Part model, mm, in its own coordinate system. A direction names the side the tool comes from. Round coordinates to 2 decimals unless told otherwise and drop trailing zeros. Loops run counter-clockwise (first coordinate to the right, second up) from the corner with the lowest first, then second, coordinate; pieces in that order, holes last. Notation, with made-up numbers: (-0.5, 14) -> (54.5, 14) arc R29 cw to (54.5, 48) -> close; hole circle Ø2 at (-29, 77.5). An arc over 180 degrees is marked (long way). Use a Markdown table: item, result. Add a question column.
Item 1: Flat gauge pins, fed straight in: pin 1 (2 mm diameter, centred on x = 0.5, z = 32.5, fed in from -Y); pin 2 (3.5 mm diameter, centred on y = -39.23, z = 96.29, fed in from -X); pin 3 (1.5 mm diameter, centred on x = 1.5, y = -72.5, fed in from +Z). Where does each tip first touch, or does it go through?
Item 2: Cut at D-D, the plane y = -136. List the corners of the cut face in (x, z).
Item 3: Cut at A-A, the plane z = 58.5. List the corners of the cut face in (x, y), plus the area to 3 significant figures.
Item 4: Probe line 1 (Y direction, x = 1.55, z = 67.5); line 2 (Z direction, x = 1, y = -125.5); line 3 (Z direction, x = 2.4, y = -58.5). List the from-to ranges inside material, lowest first. Write a range as [from, to].
Item 5: Cut at B-B, the plane y = -99. List the corners of the cut face in (x, z), plus the area to 3 significant figures.
Item 6: Cut at C-C, the plane x = 0.6. State how many separate pieces and enclosed holes the cut face has, plus the area to 3 significant figures.
Item 7: Which spindle directions (+Z, -Z, +X, -X, +Y, -Y) get a long thin tool onto all of the face, cutting with end or side? Do faces 4 (the face through (2, -186.521, 27)), 5 (the face through (2.03, -120.35, 106.77)), 6 (the face through (2, -190.521, 120)), 7 (the face through (2, -133, 10.903)), 8 (the face through (2, -188, 104.903)). Say none if no direction does.
Item 8: Two-plate mould, pull along Z, no slides. Class faces 1 (the face through (2, -186.521, 89)), 2 (the face through (2.03, -91.6, 151.05)), 3 (the face through (2, -186.521, 151)): pulls with the +Z half, pulls with the -Z half, needs draft (parallel to the pull), parting line crosses it, or undercut.
```python
from build123d import *

# Parameters (mm, degrees)
AUFSATZ_LINEAR_AUSTRAGEN1_DEPTH      = 4
SKIZZE1_9_R                          = 10
SCHNITT_LINEAR_AUSTRAGEN1_DEPTH      = 6
F_4_1_4_1_DURCHMESSER_BOHRUNG1_D     = 4.1
F_4_1_4_1_DURCHMESSER_BOHRUNG1_DEPTH = 20
F_4_1_4_1_DURCHMESSER_BOHRUNG1_TIP   = 1.231764269
FASE1_SIZE                           = 1
SCHNITT_LINEAR_AUSTRAGEN2_DEPTH      = 251.325290812
SCHNITT_LINEAR_AUSTRAGEN2_DEPTH_BACK = 10
F_4_8_4_8_DURCHMESSER_BOHRUNG1_D     = 4.8
F_4_8_4_8_DURCHMESSER_BOHRUNG1_DEPTH = 4
F_4_8_4_8_DURCHMESSER_BOHRUNG1_TIP   = 1.442065486
SKIZZE21_R                           = 37.5
SCHNITT_LINEAR_AUSTRAGEN3_DEPTH      = 251.325290812
DURCHGANGSLOCH_F_R_M41_D             = 4.5
KREISMUSTER1_COUNT                   = 6
M3_GEWINDEBOHRUNG1_D                 = 2.5
M3_GEWINDEBOHRUNG1_DEPTH             = 8.5
M3_GEWINDEBOHRUNG1_TIP               = 0.751075774
SCHNITT_LINEAR_AUSTRAGEN4_DEPTH      = 251.325290812
SCHNITT_LINEAR_AUSTRAGEN5_DEPTH      = 251.325290812
VERRUNDUNG1_R                        = 6
SKIZZE31_W                           = 4
SKIZZE31_H                           = 30
AUFSATZ_LINEAR_AUSTRAGEN2_DEPTH      = 4


with BuildPart() as part:
    # Skizze1 → Aufsatz-Linear austragen1 (new body)
    with BuildSketch(Plane(origin=(0, 0, 0), x_dir=(0, 0, -1), z_dir=(1, 0, 0))):
        with BuildLine():
            Line((-120.903454086, -13.395859459), (-120.903454086, -24.075118314))
            ThreePointArc((-120.903454086, -24.075118314), (-140.766673303, -45.238586838), (-150.337818424, -72.639919993))
            Line((-150.337818424, -72.639919993), (-166.903454086, -186.520744783))
            Line((-166.903454086, -186.520744783), (-10.903454086, -186.520744783))
            Line((-10.903454086, -186.520744783), (-1.903454086, -186.520744783))
            Line((-1.903454086, -186.520744783), (-1.903454086, -81.52074478))
            ThreePointArc((-1.903454086, -81.52074478), (-41.654250272, -12.960552248), (-120.903454086, -13.395859459))
        make_face()
    extrude(amount=AUFSATZ_LINEAR_AUSTRAGEN1_DEPTH)

    # Skizze1_9 → Schnitt-Linear austragen1 (cut)
    with BuildSketch(Plane(origin=(0, 0, 0), x_dir=(0, 0, -1), z_dir=(1, 0, 0))):
        with Locations((-80.903454086, -81.52074478)):
            Circle(SKIZZE1_9_R)
    extrude(amount=SCHNITT_LINEAR_AUSTRAGEN1_DEPTH, mode=Mode.SUBTRACT)

    # 4.1 _4.1_ Durchmesser Bohrung1
    with Locations(Plane.ZY):
        with Locations((80.903454086, -66.02074478), (96.403454086, -81.52074478), (80.903454086, -97.02074478), (65.403454086, -81.52074478)):
            Hole(F_4_1_4_1_DURCHMESSER_BOHRUNG1_D / 2, depth=F_4_1_4_1_DURCHMESSER_BOHRUNG1_DEPTH)
            with Locations((0, 0, -(F_4_1_4_1_DURCHMESSER_BOHRUNG1_DEPTH + F_4_1_4_1_DURCHMESSER_BOHRUNG1_TIP / 2))):  # 118° drill point
                Cone(0, F_4_1_4_1_DURCHMESSER_BOHRUNG1_D / 2, F_4_1_4_1_DURCHMESSER_BOHRUNG1_TIP, mode=Mode.SUBTRACT)

    # Fase1
    fase1_edges = [part.edges().sort_by_distance(p)[0] for p in [
        (4, -81.52074478, 67.453454086),
        (0, -81.52074478, 67.453454086),
        (4, -97.02074478, 82.953454086),
        (0, -97.02074478, 82.953454086),
        (4, -81.52074478, 98.453454086),
        (0, -81.52074478, 98.453454086),
        (4, -66.02074478, 82.953454086),
        (0, -66.02074478, 82.953454086),
    ]]
    chamfer(fase1_edges, length=FASE1_SIZE)

    # Skizze1_18 → Schnitt-Linear austragen2 (cut, two sides: drawn at the far end of the back side and taken through both)
    with BuildSketch(Plane(origin=(0, 0, 0), x_dir=(0, 0, -1), z_dir=(1, 0, 0)).offset(-SCHNITT_LINEAR_AUSTRAGEN2_DEPTH_BACK)):
        with BuildLine():
            ThreePointArc((-1.903454086, -81.52074478), (-41.654250272, -12.960552248), (-120.903454086, -13.395859459))
            Line((-120.903454086, -13.395859459), (-120.903454086, -24.075118314))
            ThreePointArc((-120.903454086, -24.075118314), (-48.499750594, -19.47237655), (-10.903454086, -81.52074478))
            Line((-10.903454086, -81.52074478), (-10.903454086, -186.520744783))
            Line((-10.903454086, -186.520744783), (-1.903454086, -186.520744783))
            Line((-1.903454086, -186.520744783), (-1.903454086, -81.52074478))
        make_face()
    extrude(amount=SCHNITT_LINEAR_AUSTRAGEN2_DEPTH + SCHNITT_LINEAR_AUSTRAGEN2_DEPTH_BACK, mode=Mode.SUBTRACT)

    # 4.8 _4.8_ Durchmesser Bohrung1
    with Locations(Plane(origin=(4, 0, 0), x_dir=(0, 0, -1), z_dir=(1, 0, 0))):
        with Locations((-80.903454086, -46.52074478), (-80.903454086, -116.52074478)):
            Hole(F_4_8_4_8_DURCHMESSER_BOHRUNG1_D / 2, depth=F_4_8_4_8_DURCHMESSER_BOHRUNG1_DEPTH)
            with Locations((0, 0, -(F_4_8_4_8_DURCHMESSER_BOHRUNG1_DEPTH + F_4_8_4_8_DURCHMESSER_BOHRUNG1_TIP / 2))):  # 118° drill point
                Cone(0, F_4_8_4_8_DURCHMESSER_BOHRUNG1_D / 2, F_4_8_4_8_DURCHMESSER_BOHRUNG1_TIP, mode=Mode.SUBTRACT)

    # Skizze21 → Schnitt-Linear austragen3 (cut, through all)
    with BuildSketch(Plane.YZ.offset(4)):
        with Locations(Location((-81.52074478, 80.903454086, 0), (0, 0, 270))):
            Circle(SKIZZE21_R)
    extrude(amount=-SCHNITT_LINEAR_AUSTRAGEN3_DEPTH, mode=Mode.SUBTRACT)

    # Durchgangsloch f_r M41 (through all)
    with Locations(Plane(origin=(4, 0, 0), x_dir=(0, 0, -1), z_dir=(1, 0, 0))):
        with Locations((-80.903454086, -126.52074478), (-65.512547636, -123.806912715)):
            durchgangsloch_f_r_m41 = Hole(DURCHGANGSLOCH_F_R_M41_D / 2)

    # Kreismuster1: Durchgangsloch f_r M41 ×6 about axis
    kreismuster1_axis = Axis((0, -81.52074478, 80.903454086), (1, 0, 0))
    for i in range(1, KREISMUSTER1_COUNT):
        add(durchgangsloch_f_r_m41.rotate(kreismuster1_axis, i * 360 / KREISMUSTER1_COUNT), mode=Mode.SUBTRACT)

    # M3 Gewindebohrung1
    with Locations(Plane.YZ.offset(4)):
        with Locations((-176.520744783, 14.903454086), (-126.520744783, 14.903454086), (-34.851697221, 34.234406527), (-19.501031808, 103.476783545), (-81.52074478, 14.903454086), (-73.147395695, 146.370140462), (-126.520744783, 154.133475978)):
            Hole(M3_GEWINDEBOHRUNG1_D / 2, depth=M3_GEWINDEBOHRUNG1_DEPTH)
            with Locations((0, 0, -(M3_GEWINDEBOHRUNG1_DEPTH + M3_GEWINDEBOHRUNG1_TIP / 2))):  # 118° drill point
                Cone(0, M3_GEWINDEBOHRUNG1_D / 2, M3_GEWINDEBOHRUNG1_TIP, mode=Mode.SUBTRACT)

    # Skizze29 → Schnitt-Linear austragen4 (cut, through all)
    with BuildSketch(Plane.YZ.offset(4)):
        Polygon((-106.153245921, 155.212823046), (-106.729044518, 151.254482993), (-91.885269319, 149.095238254), (-91.309470722, 153.053578307), align=None)
    extrude(amount=-SCHNITT_LINEAR_AUSTRAGEN4_DEPTH, mode=Mode.SUBTRACT)

    # Skizze30 → Schnitt-Linear austragen5 (cut, through all)
    with BuildSketch(Plane.YZ.offset(4)):
        with BuildLine():
            Line((-118.770131027, 85.231643571), (-131.223971881, 86.3430511))
            ThreePointArc((-131.223971881, 86.3430511), (-128.505375819, 98.004461252), (-123.092131269, 108.685099562))
            Line((-123.092131269, 108.685099562), (-112.837536697, 101.53131253))
            ThreePointArc((-112.837536697, 101.53131253), (-116.759218059, 93.72920946), (-118.770131027, 85.231643571))
        make_face()
    extrude(amount=-SCHNITT_LINEAR_AUSTRAGEN5_DEPTH, mode=Mode.SUBTRACT)

    # Verrundung1
    verrundung1_edges = [part.edges().sort_by_distance(p)[0] for p in [
        (2, -112.837536697, 101.53131253),
        (2, -118.770131027, 85.231643571),
    ]]
    fillet(verrundung1_edges, radius=VERRUNDUNG1_R)

    # Skizze31 → Aufsatz-Linear austragen2 (add)
    with BuildSketch(Plane.XZ.offset(186.520744783)):
        with Locations((2, 57.903454086)):
            Rectangle(SKIZZE31_W, SKIZZE31_H)
        with Locations((2, 119.903454086)):
            Rectangle(SKIZZE31_W, SKIZZE31_H)
    extrude(amount=AUFSATZ_LINEAR_AUSTRAGEN2_DEPTH)


solid = part.part
```
A:
| question | item | result |
|---|---|---|
| 1 | pin 1 | stops at y = -186.52 |
| 1 | pin 2 | passes through |
| 1 | pin 3 | stops at z = 150.43 |
| 2 | outline | (0, 10.9) -> (4, 10.9) -> (4, 159.55) -> (0, 159.55) -> close |
| 3 | outline | (0, -190.52) -> (4, -190.52) -> (4, -111.59) -> (0, -111.59) -> close; (0, -51.45) -> (4, -51.45) -> (4, -15.2) -> (0, -15.2) -> close |
| 3 | area | 461 mm^2 |
| 4 | line 1 | y = [-190.52, -124.86], [-122.75, -116.54], [-46.5, -12.82] |
| 4 | line 2 | z = [10.9, 14.18], [15.62, 64.03], [66.99, 78.9], [82.91, 85.83], [104.69, 153.41], [154.85, 158.03] |
| 4 | line 3 | z = [14.8, 39.74], [44.12, 51.3], [110.51, 117.69], [122.06, 147.01] |
| 5 | outline | (0, 10.9) -> (4, 10.9) -> (4, 47.73) -> (0, 47.73) -> close; (0, 114.08) -> (4, 114.08) -> (4, 150.13) -> (0, 150.13) -> close |
| 5 | area | 291 mm^2 |
| 6 | separate pieces | 1 |
| 6 | enclosed holes | 20 |
| 6 | area | 18,500 mm^2 |
| 7 | face 4 | -Z, +X, -X, -Y |
| 7 | face 5 | +X, -X |
| 7 | face 6 | +Z, -Z, +X, -X, -Y |
| 7 | face 7 | -Z, +X, -X, +Y, -Y |
| 7 | face 8 | +X, -X, -Y |
| 8 | face 1 | undercut |
| 8 | face 2 | pulls with the +Z half |
| 8 | face 3 | needs draft |
